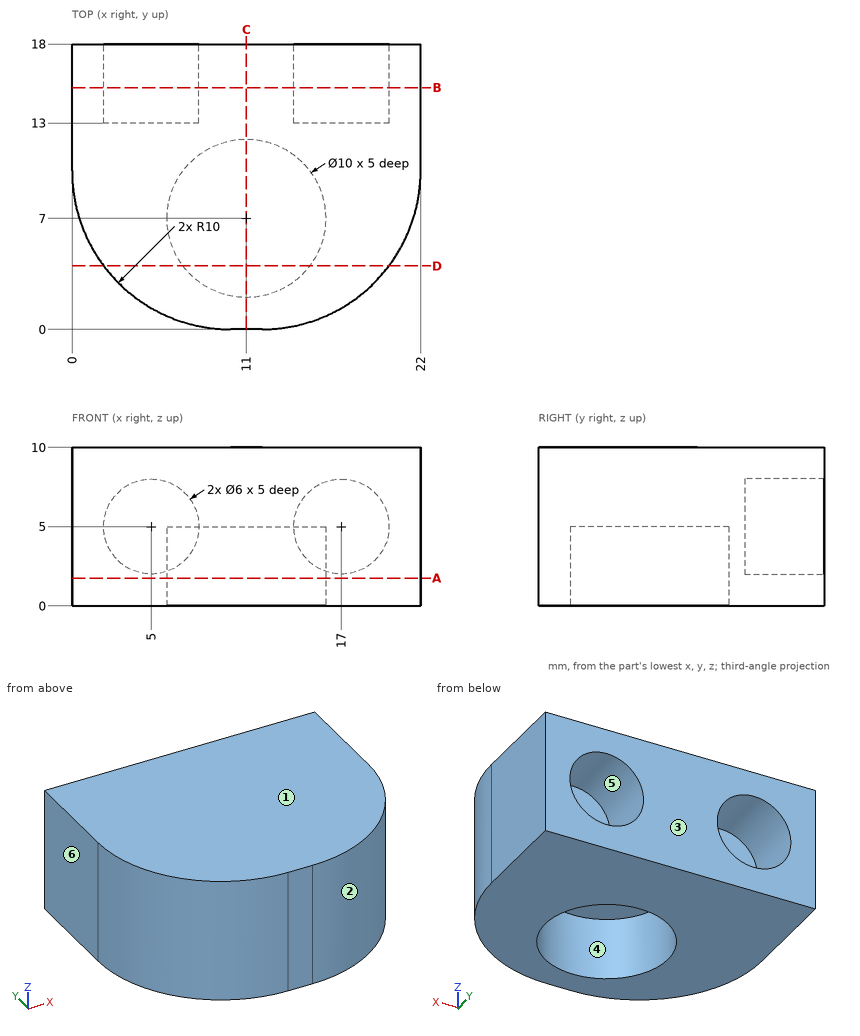
Could you check a few things on this drawing? It's one solid part, dimensions in mm from its lowest x, y, z. A direction names the side the tool comes from. Round coordinates to 2 decimals unless told otherwise and drop trailing zeros. Order: outer loops, then holes, each group sorted by start corner. A loop starts at its lowest first (then second) coordinate and runs counter-clockwise, first axis right, second up. Notation, with made-up numbers: M 76.25,33 L 88.25,33 A4 cw 88.25,38 Z; hole C -22,74 d2. An arc over 180 degrees is marked long. Use a Markdown table: item, result.
1) On a 3-axis mill with a long thin cutter (end or side, diameter ignored), from which of +Z, -Z, +X, -X, +Y, -Y can I reach the whole of each face in a straight line? I mean the marked faces 5 and 6. Say none if no direction works.
Geometry says:
| item | result |
|---|---|
| face 5 | +Y |
| face 6 | +Z, -Z, -X, +Y, -Y |
2) Imagine slicing it at A-A (z = 1.75). List the corners of the cut face in (x, y) for me, then the cut area to 3 significant figures.
Geometry says:
| item | result |
|---|---|
| outline | M 0,10 A10 ccw 10,0 L 12,0 A10 ccw 22,10 L 22,18 L 0,18 Z; hole C 11,7 d10 |
| area | 275 mm² |
3) Imagine slicing it at C-C (x = 11). List the corners of the cut face in (y, z) for me, then the cut area to 3 significant figures.
Geometry says:
| item | result |
|---|---|
| outline | M 0,0 L 2,0 L 2,5 L 12,5 L 12,0 L 18,0 L 18,10 L 0,10 Z |
| area | 130 mm² |
4) I'm going to push flat-ended pins straight in: P1, Ø4, axis at x = 7.5, z = 5.5, coming from the -Y side; P2, Ø1.5, axis at x = 7, z = 6, coming from the -Y side; P3, Ø3, axis at y = 4.5, z = 6, coming from the +X side. Where does each tip first touch, or does it pass through?
Geometry says:
| item | result |
|---|---|
| P1 | stops at y = 0.01 |
| P2 | stops at y = 0.26 |
| P3 | stops at x = 21.17 |
5) If I drill on line 1 along X through (y, z) = (16.35, 5); line 2 along X through (y, z) = (15.75, 6.25); line 3 along Y through (x, z) = (11, 2), over which ranges is the centre line in solid material (lowest first)?
Geometry says:
| item | result |
|---|---|
| line 1 | x = 0 to 2, 8 to 14, 20 to 22 |
| line 2 | x = 0 to 2.27, 7.73 to 14.27, 19.73 to 22 |
| line 3 | y = 0 to 2, 12 to 18 |
6) Imagine slicing it at B-B (y = 15.25). List the corners of the cut face in (x, z) for me.
Geometry says:
| item | result |
|---|---|
| outline | M 0,0 L 22,0 L 22,10 L 0,10 Z; hole C 5,5 d6; hole C 17,5 d6 |
7) If we mould it in two halves opening along Y, with no side actions, what happens to the marked faces 1, 2, 3 and 4? For each: +Y half, -Y half, draft (parallel to the pull), parting line (faces both ways), or undercut.
Geometry says:
| item | result |
|---|---|
| face 1 | draft |
| face 2 | -Y half |
| face 3 | +Y half |
| face 4 | undercut |
8) Imagine slicing it at D-D (y = 4). List the corners of the cut face in (x, z) for me, then the cut area to 3 significant figures.
Geometry says:
| item | result |
|---|---|
| outline | M 2,0 L 7,0 L 7,5 L 15,5 L 15,0 L 20,0 L 20,10 L 2,10 Z |
| area | 140 mm² |
